Build history of the part. All positions in model axes, mm. A direction names the side the tool comes from. Give positions to 0.01 mm unless a question says otherwise; leave off trailing zeros. Order: outer loops, then holes, each group sorted by start corner. A loop starts at its lowest first (then second) coordinate and runs counter-clockwise, first axis right, second up. Notation, with made-up numbers: (-34, 62.25) - (-5, 62.25) arc R26 ccw to (-5, 85.25) - close; hole circle Ø7 at (-34, 63.25). An arc over 180 degrees is marked (long way). One line per item, written item: value.
```python
from build123d import *

# Parameters (mm, degrees)
F1_DEPTH = 66.5
F2_R     = 1.5
F2_R_2   = 2
F2_R_3   = 0.75
F3_DEPTH = 25
F4_R     = 1.5
F5_DEPTH = 25
F6_R     = 1
F7_DEPTH = 25
F8_R     = 1.5
F9_DEPTH = 1.5


with BuildPart() as f1:
    # F0 (on Top) → F1 (new body)
    with BuildSketch(Plane.XY):
        with BuildLine():
            Line((-64.5, -33), (-64.5, 33))
            Line((-64.5, 33), (-66, 33))
            Line((-66, 33), (-66, -33))
            ThreePointArc((-66, -33), (-64.535534, -36.535534), (-61, -38))
            Line((-61, -38), (51, -38))
            ThreePointArc((51, -38), (54.535534, -36.535534), (56, -33))
            Line((56, -33), (56, 33))
            ThreePointArc((56, 33), (54.535534, 36.535534), (51, 38))
            Line((51, 38), (-46.5, 38))
            ThreePointArc((-46.5, 38), (-50.035534, 36.535534), (-51.5, 33))
            Line((-51.5, 33), (-51.5, 0))
            Line((-51.5, 0), (-50, 0))
            Line((-50, 0), (-50, 33))
            ThreePointArc((-50, 33), (-48.974874, 35.474874), (-46.5, 36.5))
            Line((-46.5, 36.5), (51, 36.5))
            ThreePointArc((51, 36.5), (53.474874, 35.474874), (54.5, 33))
            Line((54.5, 33), (54.5, -33))
            ThreePointArc((54.5, -33), (53.474874, -35.474874), (51, -36.5))
            Line((51, -36.5), (-61, -36.5))
            ThreePointArc((-61, -36.5), (-63.474874, -35.474874), (-64.5, -33))
        make_face()
    extrude(amount=F1_DEPTH)

    # F2 (on face) → F3 (cut)
    with BuildSketch(Plane.XZ.offset(38)):
        with BuildLine():
            Line((22, 52.25), (-22, 52.25))
            ThreePointArc((-22, 52.25), (-24.12132, 51.37132), (-25, 49.25))
            Line((-25, 49.25), (-25, 17.25))
            ThreePointArc((-25, 17.25), (-24.12132, 15.12868), (-22, 14.25))
            Line((-22, 14.25), (22, 14.25))
            ThreePointArc((22, 14.25), (24.12132, 15.12868), (25, 17.25))
            Line((25, 17.25), (25, 49.25))
            ThreePointArc((25, 49.25), (24.12132, 51.37132), (22, 52.25))
        make_face()
        with Locations((-29, 33.25)):
            Circle(F2_R)
        with Locations((29, 33.25)):
            Circle(F2_R)
        with Locations((-25, 58.25)):
            Circle(F2_R_2)
        with Locations((25, 58.25)):
            Circle(F2_R_2)
        with Locations((-25, 8.25)):
            Circle(F2_R_2)
        with Locations((25, 8.25)):
            Circle(F2_R_2)
        with BuildLine():
            ThreePointArc((-7.5, 8.75), (-7.06066, 7.68934), (-6, 7.25))
            Line((-6, 7.25), (6, 7.25))
            ThreePointArc((6, 7.25), (7.06066, 7.68934), (7.5, 8.75))
            ThreePointArc((7.5, 8.75), (7.06066, 9.81066), (6, 10.25))
            Line((6, 10.25), (-6, 10.25))
            ThreePointArc((-6, 10.25), (-7.06066, 9.81066), (-7.5, 8.75))
        make_face()
        with Locations((-10.5, 8.75)):
            Circle(F2_R_3)
        with Locations((10.5, 8.75)):
            Circle(F2_R_3)
        with Locations((-19, 8.25)):
            Circle(F2_R_2)
        with Locations((-19, 58.25)):
            Circle(F2_R_2)
        with Locations((19, 58.25)):
            Circle(F2_R_2)
        with Locations((16, 8.25)):
            Circle(F2_R_2)
    extrude(amount=-F3_DEPTH, mode=Mode.SUBTRACT)

    # F4 (on face) → F5 (cut)
    with BuildSketch(Plane(origin=(0, 38, 0), x_dir=(-1, 0, 0), z_dir=(0, 1, 0))):
        with Locations((-41, 57)):
            Circle(F4_R)
        with Locations((-41, 9)):
            Circle(F4_R)
        with Locations((41, 9)):
            Circle(F4_R)
        with Locations((41, 57)):
            Circle(F4_R)
        with Locations((41, 16.375)):
            Circle(F4_R)
        with Locations((41, 49.625)):
            Circle(F4_R)
    extrude(amount=-F5_DEPTH, mode=Mode.SUBTRACT)

    # F6 (on face) → F7 (cut)
    with BuildSketch(Plane.YZ.offset(56)):
        with BuildLine():
            Line((-17, 58.5), (-21, 58.5))
            ThreePointArc((-21, 58.5), (-23.12132, 57.62132), (-24, 55.5))
            Line((-24, 55.5), (-24, 11))
            ThreePointArc((-24, 11), (-23.12132, 8.87868), (-21, 8))
            Line((-21, 8), (-17, 8))
            ThreePointArc((-17, 8), (-14.87868, 8.87868), (-14, 11))
            Line((-14, 11), (-14, 55.5))
            ThreePointArc((-14, 55.5), (-14.87868, 57.62132), (-17, 58.5))
        make_face()
        with BuildLine():
            Line((24, 58.5), (-5, 58.5))
            ThreePointArc((-5, 58.5), (-7.12132, 57.62132), (-8, 55.5))
            Line((-8, 55.5), (-8, 11))
            ThreePointArc((-8, 11), (-7.12132, 8.87868), (-5, 8))
            Line((-5, 8), (24, 8))
            ThreePointArc((24, 8), (26.12132, 8.87868), (27, 11))
            Line((27, 11), (27, 55.5))
            ThreePointArc((27, 55.5), (26.12132, 57.62132), (24, 58.5))
        make_face()
        with Locations((-19, 61.5)):
            Circle(F6_R)
        with Locations((9.5, 61.5)):
            Circle(F6_R)
        with Locations((9.5, 5)):
            Circle(F6_R)
        with Locations((-19, 5)):
            Circle(F6_R)
    extrude(amount=-F7_DEPTH, mode=Mode.SUBTRACT)

    # F8 (on face) → F9 (cut)
    with BuildSketch(Plane(origin=(-66, 0, 0), x_dir=(0, -1, 0), z_dir=(-1, 0, 0))):
        with Locations((8.5, 57.25)):
            Circle(F8_R)
        with Locations((8.5, 9.25)):
            Circle(F8_R)
    extrude(amount=-F9_DEPTH, mode=Mode.SUBTRACT)


solid = f1.part
```
(1) Drill centre lines: line 1 (X direction, y = 28.5, z = 49); line 2 (X direction, y = 10.5, z = 48.5); line 3 (Y direction, x = -24.5, z = 13.5). Where is each one in solid material? Low to high.
Completed:
line 1: -66 to -64.5, -51.5 to -50, 54.5 to 56
line 2: -66 to -64.5, -51.5 to -50
line 3: -38 to -36.5, 36.5 to 38
(2) Pull direction Z, two halves, no side cores. Call faces 1 (the face through (55.26, -23.1, 57.64)), 2 (the face through (-63.45, -35.5, 32.78)), 3 (the face through (55.26, 26.1, 8.86)), 4 (the face through (-14, 37, 0)): +Z half, -Z half, draft (parallel to the pull), parting line (faces both ways), or undercut.
Completed:
face 1: undercut
face 2: draft
face 3: undercut
face 4: -Z half
(3) Slice it at C-C, the plane y = -27.5. Give the cut face in (x, z), and give its area (4 significant figures).
Completed:
outline: (-66, 0) - (-64.5, 0) - (-64.5, 66.5) - (-66, 66.5) - close; (54.5, 0) - (56, 0) - (56, 66.5) - (54.5, 66.5) - close
area: 199.5 mm²
(4) Slice it at B-B, the plane x = 29. Give the cut face in (y, z), and give its area (3 significant figures).
Completed:
outline: (-38, 0) - (-36.5, 0) - (-36.5, 31.75) - (-38, 31.75) - close; (-38, 34.75) - (-36.5, 34.75) - (-36.5, 66.5) - (-38, 66.5) - close; (36.5, 0) - (38, 0) - (38, 66.5) - (36.5, 66.5) - close
area: 195 mm²
(5) Slice it at D-D, the plane y = 12.5. Give the cut face in (x, z).
Completed:
outline: (-66, 0) - (-64.5, 0) - (-64.5, 66.5) - (-66, 66.5) - close; (-51.5, 0) - (-50, 0) - (-50, 66.5) - (-51.5, 66.5) - close; (54.5, 0) - (56, 0) - (56, 8) - (54.5, 8) - close; (54.5, 58.5) - (56, 58.5) - (56, 66.5) - (54.5, 66.5) - close
(6) Pin check, flat tips, straight feed: P1, Ø3.5, axis at x = -19, z = 8.25, coming from the -Y side; P2, Ø3, axis at y = -1, z = 32, coming from the +X side. Stop position of each tip, or through.
Completed:
P1: y = 36.5
P2: x = -50
(7) Slice it at A-A, the plane z = 25. Count the separate pieces of the cut face and the enclosed holes in it, and give its area (3 significant figures).
Completed:
separate pieces: 4
enclosed holes: 0
area: 459 mm²
(8) 3-axis set-ups, long thin cutter, end or side, ignore diameter. For faces 5 (the face through (55.26, -14.86, 57.6)), 6 (the face through (18.74, -37.26, 60.233)), 7 (the face through (42.11, 37.26, 58.01)), 8 (the face through (-49, 35.45, 32.78)): which of +Z, -Z, +X, -X, +Y, -Y reach the whole face in a straight line?
Completed:
face 5: +X
face 6: -Y
face 7: +Y
face 8: +Z, -Z
